```python
from build123d import *

# Parameters (mm, degrees)
F0_W     = 22
F0_H     = 24.8139590786
F1_DEPTH = 10
F2_R     = 8
F3_DEPTH = 20
F4_R     = 4
F5_DEPTH = 47
F6_R     = 2.99999


# Not quite as in the source:
# - a fillet or chamfer is up to 0.001 mm smaller than in the source, because OpenCascade refuses the exact size


with BuildPart() as f1:
    # F0 (on Top) → F1 (new body)
    with BuildSketch(Plane.XY):
        Rectangle(F0_W, F0_H)
    extrude(amount=F1_DEPTH)

    # F2 (on face) → F3 (join)
    with BuildSketch(Plane.XY.offset(10)):
        Circle(F2_R)
    extrude(amount=F3_DEPTH)

    # F4 (on face) → F5 (join)
    with BuildSketch(Plane.XY.offset(30)):
        Circle(F4_R)
    extrude(amount=F5_DEPTH)

    # F6 (radius 3 in the source; OpenCascade refuses exactly that, so slightly less here)
    f6_edges = [f1.edges().sort_by_distance(p)[0] for p in [
        (8, 0, 20),
        (-8, 0, 10),
        (-8, 0, 30),
    ]]
    fillet(f6_edges, radius=F6_R)


solid = f1.part
```
Read the model definition and answer for the solid it produces. Units are mm, in the model's axes. A direction names the side the tool comes from. Coordinates: 2 decimals unless noted, no trailing zeros. Write each loop counter-clockwise with the first axis right and the second up, starting at its lowest first coordinate (ties: lowest second). Pieces come first, ordered by that corner, then holes. Notation, with made-up numbers: (70, 43) -> (86, 43) arc R19 cw to (86, 71) -> close; hole circle Ø4 at (-34, 62.5). An arc over 180 degrees is marked (long way). Write item = value, one per line.
(1) Straight lines are drawn through the part: L1, parallel to Z at x = -2.25, y = -4.25; L2, parallel to Z at x = 4.75, y = -10.5; L3, parallel to X at y = 2.5, z = 14. For each, find the intervals that lie inside material, in ascending order. Write a range as from..to.
From the geometry:
L1 = 0..30
L2 = 0..10
L3 = -7.6..7.6
(2) Section B-B on x = 0 is taken. Write down the section's boundary in (y, z), plus the area to 3 significant figures.
From the geometry:
outline = (-12.41, 0) -> (12.41, 0) -> (12.41, 10) -> (11, 10) arc R3 cw to (8, 13) -> (8, 27) arc R3 ccw to (5, 30) -> (4, 30) -> (4, 77) -> (-4, 77) -> (-4, 30) -> (-5, 30) arc R3 ccw to (-8, 27) -> (-8, 13) arc R3 cw to (-11, 10) -> (-12.41, 10) -> close
area = 944 mm2
(3) Section C-C on z = 67 is taken. Write down the section's boundary in (x, y), plus the area to 3 significant figures.
From the geometry:
outline = circle Ø8 at (0, 0)
area = 50.3 mm2
(4) Which of the six approach directions +Z, -Z, +X, -X, +Y, -Y give full straight-line access (tool end or side, diameter ignored) to faces 1 (the face through (0, -12.407, 5)), 2 (the face through (-1.73, -7.81, 19.9))?
From the geometry:
face_1 = +Z, -Z, +X, -X, -Y
face_2 = +Z
(5) Given pin 1 Ø1.5 at (x, y) = (-1, 2.5) entering from -Z; pin 2 Ø8 at (y, z) = (-3.5, 69) entering from +X; pin 3 Ø10 at (x, z) = (-7, 26.5) entering from +Y; pin 4 Ø1.5 at (x, y) = (4, 4.5) entering from +Z, each flat-ended and moving along its own axis, determine where each tip first touches the part or whether it passes through.
From the geometry:
pin_1 = 0
pin_2 = 4
pin_3 = 7.75
pin_4 = 29.99
